Drawing for the job (mm, zero at the part's lowest x, y, z). A direction names the side the tool comes from. Coordinates: 2 decimals unless noted, no trailing zeros. Write each loop counter-clockwise with the first axis right and the second up, starting at its lowest first coordinate (ties: lowest second). Pieces come first, ordered by that corner, then holes. Notation, with made-up numbers: M -17,78.5 L -13,78.5 A23 cw -13,96.5 Z; hole C 89,25.25 d5. An arc over 180 degrees is marked long. Use a Markdown table: item, result. Add a question column.
Q1. Slice it at C-C on y = 37.5. Write the cut outline in (x, z) (1 decimal), then the cut area to 3 significant figures.
Q2. Slice it at B-B on x = 88. Write the cut outline in (y, z) (1 decimal).
Q3. Slice it at A-A on z = 42. Write the cut outline in (x, y), then the cut area to 3 significant figures.
Q4. Wall check: L1, parallel to X at y = 56.5, z = 49 (1 decimal); L2, parallel to X at y = 4, z = 21 (1 decimal); L3, parallel to Y at x = 55.5, z = 92.5. Give the ranges that are in metal, low to high. Write a range as from..to.
Q5. Pin check, flat tips, straight feed: pin 1 Ø2 at (x, y) = (93, 12) entering from -Z (1 decimal); pin 2 Ø8 at (y, z) = (28.5, 61) entering from -X; pin 3 Ø4 at (x, y) = (92, 18.5) entering from -Z (1 decimal); pin 4 Ø8 at (y, z) = (18.5, 27.5) entering from -X. Stop position of each tip, or through.
Q6. Tool access for the marked faces 1 and 2: list every direction of +Z, -Z, +X, -X, +Y, -Y with a clear straight run to the whole face (end or side of a thin tool).
Q7. Slice it at D-D on z = 8. Write the cut outline in (x, y) (1 decimal), then the cut area to 3 significant figures.
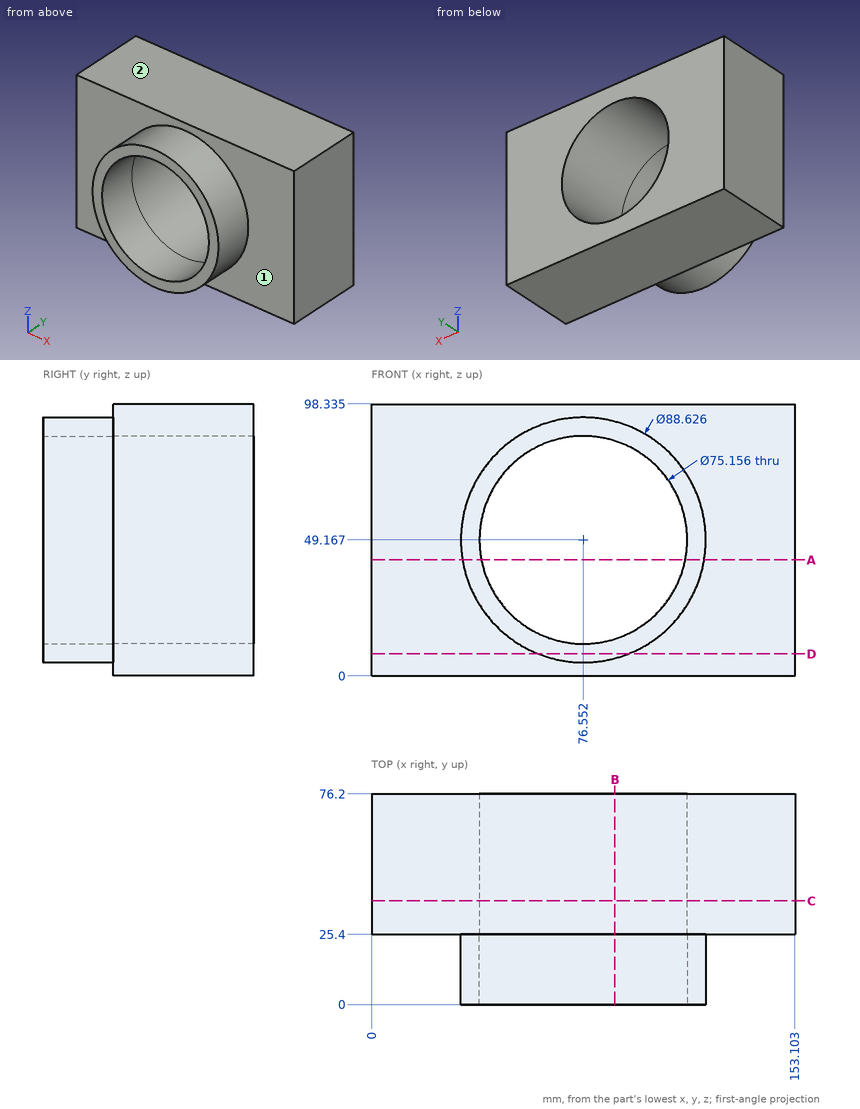
Recorded:
| question | item | result |
|---|---|---|
| 1 | outline | M 0,0 L 153.1,0 L 153.1,98.3 L 0,98.3 Z; hole C 76.6,49.2 d75.2 |
| 1 | area | 10,600 mm² |
| 2 | outline | M 0,6.4 L 25.4,6.4 L 25.4,0 L 76.2,0 L 76.2,13.4 L 0,13.4 Z; M 0,85 L 76.2,85 L 76.2,98.3 L 25.4,98.3 L 25.4,92 L 0,92 Z |
| 3 | outline | M 0,25.4 L 32.82,25.4 L 32.82,0 L 39.66,0 L 39.66,76.2 L 0,76.2 Z; M 113.44,0 L 120.28,0 L 120.28,25.4 L 153.1,25.4 L 153.1,76.2 L 113.44,76.2 Z |
| 3 | area | 4,380 mm² |
| 4 | L1 | 0..39, 114.1..153.1 |
| 4 | L2 | 42.3..51.7, 101.4..110.8 |
| 4 | L3 | 25.4..76.2 |
| 5 | pin 1 | z = 7.6 |
| 5 | pin 2 | x = 0 |
| 5 | pin 3 | z = 6.9 |
| 5 | pin 4 | x = 35.91 |
| 6 | face 1 | -Y |
| 6 | face 2 | +Z, +X, -X, +Y, -Y |
| 7 | outline | M 0,25.4 L 60.2,25.4 L 60.2,0 L 92.9,0 L 92.9,25.4 L 153.1,25.4 L 153.1,76.2 L 0,76.2 Z |
| 7 | area | 8,610 mm² |
